Autodesk Inventor part; units mm, degrees
ref_plane "XZ Plane" through (0, 0, 0) normal (0, 1, 0) x (-1, 0, 0)
ref_plane "XY Plane" through (0, 0, 0) normal (0, 0, 1) x (1, 0, 0)
sketch "Sketch1" plane through (0, 0, 0) normal (0, 0, 1) x (1, 0, 0)
  line L0 (-19.05, -25.4) -> (19.05, -25.4)
  line L1 (19.05, -25.4) -> (19.05, 25.4)
  line L2 (19.05, 25.4) -> (-19.05, 25.4)
  line L3 (-19.05, 25.4) -> (-19.05, -25.4)
  line L4 (-19.05, -25.4) -> (19.05, 25.4) construction
  line L5 (19.05, -25.4) -> (-19.05, 25.4) construction
  point P0 (0, 0)
  dimension "d0" = 38.1
  dimension "d1" = 50.8
extrude "Extrusion1" add sketch "Sketch1" along normal mid plane 19.05
sketch "Sketch2" plane through (-19.05, 25.4, 9.525) normal (0, 1, 0) x (1, 0, 0)
  line L0 (34.925, 3.175) -> (34.925, 15.875)
  line L1 (34.925, 15.875) -> (3.175, 15.875)
  line L2 (3.175, 15.875) -> (3.175, 3.175)
  line L3 (3.175, 3.175) -> (34.925, 3.175)
  line L4 (34.925, 3.175) -> (3.175, 15.875) construction
  line L5 (34.925, 15.875) -> (3.175, 3.175) construction
  line L6 (0, 19.05) -> (38.1, 19.05)
  line L7 (0, 19.05) -> (0, 0)
  point P0 (19.05, 9.525)
  dimension "d4" = 3.175
  dimension "d5" = 3.175
extrude "Extrusion2" cut sketch "Sketch2" against normal through all
properties part number "magnetHolder" material "Aluminum 6061"
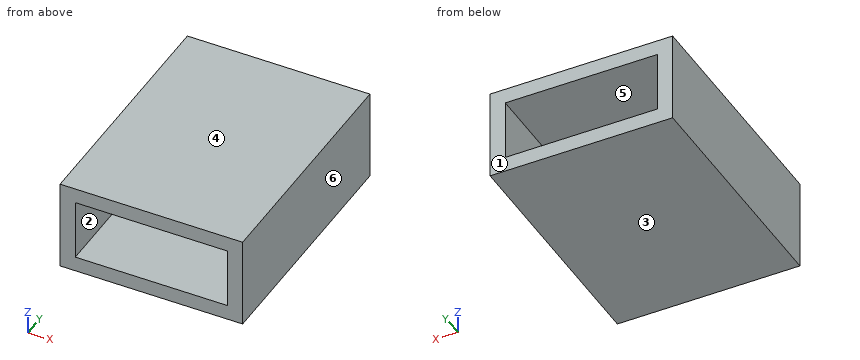
Can you work these out from the model? Positions are in its coordinate system, mm. Face numbers are marked on the shaded views. A direction names the side the tool comes from. Coordinates: 2 decimals unless noted, no trailing zeros. Write each loop counter-clockwise with the first axis right and the second up, starting at its lowest first coordinate (ties: lowest second). Pieces come first, ordered by that corner, then holes. Notation, with made-up numbers: M -16.75,68 L -9.75,68 A26 cw -9.75,95 Z; hole C -7,-8.75 d7. An arc over 180 degrees is marked long. Use one line per item in the form item = value.
Q1. I need wall thicknesses on line 1 along X through (y, z) = (-9, -4.75) (3 decimals); line 2 along Z through (x, y) = (-6.5, -22) (3 decimals). Which ranges of each line are inside material? Lowest first, please. Write a range as from..to.
Model answer:
line_1 = -19.05..-15.875, 15.875..19.05
line_2 = -9.525..-6.35, 6.35..9.525
Q2. If we section it at C-C (y = -2): Write out the boundary of the cut face in (x, z) (3 decimals), then the cut area to 3 significant figures.
Model answer:
outline = M -19.05,-9.525 L 19.05,-9.525 L 19.05,9.525 L -19.05,9.525 Z; hole M -15.875,-6.35 L 15.875,-6.35 L 15.875,6.35 L -15.875,6.35 Z
area = 323 mm^2
Q3. For the marked faces 1 and 2, which set-ups out of +Z, -Z, +X, -X, +Y, -Y let a thin tool reach every point of the face, with its end or its side?
Model answer:
face_1 = +Z, -Z, +X, -X, +Y
face_2 = +Y, -Y
Q4. If we section it at A-A (x = -7): Write out the boundary of the cut face in (y, z) (3 decimals).
Model answer:
outline = M -25.4,-9.525 L 25.4,-9.525 L 25.4,-6.35 L -25.4,-6.35 Z; M -25.4,6.35 L 25.4,6.35 L 25.4,9.525 L -25.4,9.525 Z
Q5. If we section it at B-B (z = 2.5): Write out the boundary of the cut face in (x, y) (3 decimals), then the cut area to 3 significant figures.
Model answer:
outline = M -19.05,-25.4 L -15.875,-25.4 L -15.875,25.4 L -19.05,25.4 Z; M 15.875,-25.4 L 19.05,-25.4 L 19.05,25.4 L 15.875,25.4 Z
area = 323 mm^2
Q6. We'd pull the mould along Z, two halves only. Please class the marked faces 3, 4, 5 and 6: +Z half, -Z half, draft (parallel to the pull), parting line (faces both ways), or undercut.
Model answer:
face_3 = -Z half
face_4 = +Z half
face_5 = undercut
face_6 = draft
